For this review, use the dimensioned drawing (mm, ordinates from the lowest corner) and the shaded views. Coordinates: 2 decimals unless noted, no trailing zeros. Order: outer loops, then holes, each group sorted by start corner. A loop starts at its lowest first (then second) coordinate and runs counter-clockwise, first axis right, second up. Notation, with made-up numbers: (-6, 5.25) -> (42, 5.25) arc R25 cw to (42, 37.25) -> close; hole circle Ø10 at (57.5, 82). An arc over 180 degrees is marked (long way). Return JSON: item names as keys, results as strings. Group by question number.
Item 1: Take a section at A-A (y = 117.5). Write out the cut boundary in (x, z), then the cut area to 3 significant figures.
Item 2: For line 1 along Y through (x, z) = (95, 0.55); line 2 along Y through (x, z) = (112.5, 0.9); line 3 along X through (y, z) = (110, 0.65), list the stretches that pass through material, from the lowest coordinate up.
Item 3: Take a section at B-B (x = 112.5). Write out the cut boundary in (y, z), then the cut area to 3 significant figures.
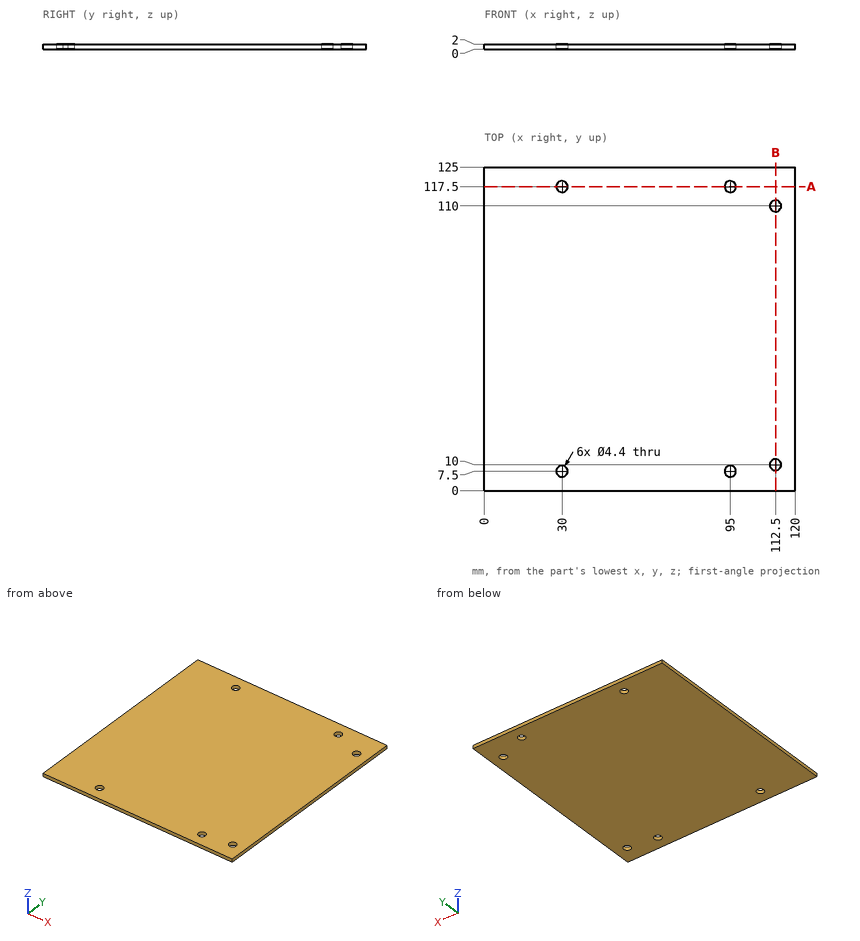
Findings below:
{
 "1": {"outline": "(0, 0) -> (27.8, 0) -> (27.8, 2) -> (0, 2) -> close; (32.2, 0) -> (92.8, 0) -> (92.8, 2) -> (32.2, 2) -> close; (97.2, 0) -> (120, 0) -> (120, 2) -> (97.2, 2) -> close", "area": "222 mm2"},
 "2": {"line 1": "y = 0 to 5.3, 9.7 to 115.3, 119.7 to 125", "line 2": "y = 0 to 7.8, 12.2 to 107.8, 112.2 to 125", "line 3": "x = 0 to 110.3, 114.7 to 120"},
 "3": {"outline": "(0, 0) -> (7.8, 0) -> (7.8, 2) -> (0, 2) -> close; (12.2, 0) -> (107.8, 0) -> (107.8, 2) -> (12.2, 2) -> close; (112.2, 0) -> (125, 0) -> (125, 2) -> (112.2, 2) -> close", "area": "232 mm2"}
}
